Design review of the part built by this model. Coordinates are the model's own, in mm. A direction names the side the tool comes from. Round coordinates to 2 decimals unless told otherwise and drop trailing zeros. Order: outer loops, then holes, each group sorted by start corner. A loop starts at its lowest first (then second) coordinate and runs counter-clockwise, first axis right, second up. Notation, with made-up numbers: M -38.5,74 L 4.5,74 A24 ccw 4.5,90 Z; hole C -6.75,76.25 d5. An arc over 180 degrees is marked long. Write each question's results on one line, items separated by ' | '. Start each with the question number.
Item 1: Wall thickness on line 1 (Y direction, x = 0, z = 31); line 2 (X direction, y = 14, z = 9.5); line 3 (Z direction, x = 25, y = -6): over which ranges is each line inside the solid? List them lowest first. Write a range as [from, to].
Item 2: Clearance check with flat-ended pins moving along their axes: pin 1 (4 mm diameter, centred on x = -21, z = 13, fed in from +Y); pin 2 (1.5 mm diameter, centred on x = 18.5, z = 8.5, fed in from +Y); pin 3 (6.5 mm diameter, centred on x = 20.57, y = -11.88, fed in from +Z). State where each tip first meets the part, or that it passes through.
Item 3: Machinability: for faces 4 (the flat face through (12, -12, 0)), 5 (the cylindrical face through (21.722, 14.093, 7.395)), 6 (the flat face through (12, -12, 15)), which of the approach directions +Z, -Z, +X, -X, +Y, -Y give a long, thin tool a straight path to every point of the face, cutting with its end or side? Answer none if there is none.
Item 4: The part is to be moulded in two halves that separate along Y. For faces 1 (the cylindrical face through (21.722, -9.657, 7.395)), 2 (the cylindrical face through (-14.985, -0.66, 16.479)), 3 (the flat face through (6.5, -6.5, 18)), say which applies: +Y half, -Y half, draft (parallel to the pull), parting line (faces both ways), or undercut.
Item 5: Take a section at B-B, the plane y = 0. Write out the cut boundary in (x, z), plus the area to 3 significant figures.
Item 6: Take a section at D-D, the plane x = -10.5. Write out the cut boundary in (y, z).
Item 7: Take a section at A-A, the plane x = 0. Write out the cut boundary in (y, z), plus the area to 3 significant figures.
Item 8: Take a section at C-C, the plane z = 8. Write out the cut boundary in (x, y) (3 decimals), plus the area to 3 significant figures.
Autodesk Inventor part; units mm, degrees
ref_plane "YZ Plane" through (0, 0, 0) normal (1, 0, 0) x (0, 1, 0)
ref_plane "XZ Plane" through (0, 0, 0) normal (0, 1, 0) x (-1, 0, 0)
ref_plane "XY Plane" through (0, 0, 0) normal (0, 0, 1) x (1, 0, 0)
sketch "Sketch1" plane through (0, 0, 0) normal (0, 0, 1) x (1, 0, 0)
  circle A0 centre (0, 0) radius 28
  line L0 (0, 0) -> (0, 23.75)
  circle A1 centre (0, 23.75) radius 2.5
  circle A2 centre (-20.5681, 11.875) radius 2.5
  circle A3 centre (-20.5681, -11.875) radius 2.5
  circle A4 centre (0, -23.75) radius 2.5
  circle A5 centre (20.5681, -11.875) radius 2.5
  circle A6 centre (20.5681, 11.875) radius 2.5
  dimension "d3" = 56
  dimension "d4" = 23.75
  dimension "d5" = 5
  dimension "d6" = 360
extrude "Extrusion1" add sketch "Sketch1" along normal blind 15
sketch "Sketch2" plane through (0, 0, 15) normal (0, 0, 1) x (1, 0, 0)
  circle A0 centre (0, 0) radius 15
  dimension "d9" = 30
extrude "Extrusion2" add sketch "Sketch2" along normal blind 3
sketch "Sketch3" plane through (0, 0, 18) normal (0, 0, 1) x (1, 0, 0)
  circle A0 centre (0, 0) radius 8.5
  dimension "d12" = 17
extrude "Extrusion3" add sketch "Sketch3" along normal blind 18
sketch "Sketch4" plane through (0, 0, 36) normal (0, 0, 1) x (1, 0, 0)
  circle A0 centre (0, 0) radius 4
  dimension "d15" = 8
extrude "Extrusion4" cut sketch "Sketch4" against normal through all
sketch "Sketch5" plane through (0, 0, 0) normal (0, 0, -1) x (-1, 0, 0)
  circle A0 centre (0, 0) radius 15
  circle A1 centre (0, 0) radius 4
  dimension "d18" = 30
extrude "Extrusion5" add sketch "Sketch5" along normal blind 3
properties part number "HubOmni1" material "Iron, Cast"
Results list:
1) line 1: [-8.5, -4], [4, 8.5] | line 2: [-24.25, -21.89], [-19.25, 19.25], [21.89, 24.25] | line 3: [0, 15]
2) pin 1: y = 20.57 | pin 2: y = 21.65 | pin 3: z = 15
3) face 4: -Z | face 5: +Z, -Z | face 6: +Z
4) face 1: undercut | face 2: parting line | face 3: draft
5) outline: M -28,0 L -15,0 L -15,-3 L -4,-3 L -4,36 L -8.5,36 L -8.5,18 L -15,18 L -15,15 L -28,15 Z; M 4,-3 L 15,-3 L 15,0 L 28,0 L 28,15 L 15,15 L 15,18 L 8.5,18 L 8.5,36 L 4,36 Z | area: 1,010 mm²
6) outline: M -25.96,0 L -10.71,0 L -10.71,-3 L 10.71,-3 L 10.71,0 L 25.96,0 L 25.96,15 L 10.71,15 L 10.71,18 L -10.71,18 L -10.71,15 L -25.96,15 Z
7) outline: M -28,0 L -26.25,0 L -26.25,15 L -28,15 Z; M -21.25,0 L -15,0 L -15,-3 L -4,-3 L -4,36 L -8.5,36 L -8.5,18 L -15,18 L -15,15 L -21.25,15 Z; M 4,-3 L 15,-3 L 15,0 L 21.25,0 L 21.25,15 L 15,15 L 15,18 L 8.5,18 L 8.5,36 L 4,36 Z; M 26.25,0 L 28,0 L 28,15 L 26.25,15 Z | area: 864 mm²
8) outline: C 0,0 d56; hole C -20.568,-11.875 d5; hole C -20.568,11.875 d5; hole C 0,0 d8; hole C 0,-23.75 d5; hole C 0,23.75 d5; hole C 20.568,-11.875 d5; hole C 20.568,11.875 d5 | area: 2,290 mm²
